The model under review builds one solid part; all positions refer to its coordinate system, in mm. Give positions to 0.01 mm unless a question says otherwise; leave off trailing zeros. Order: outer loops, then holes, each group sorted by start corner. A loop starts at its lowest first (then second) coordinate and runs counter-clockwise, first axis right, second up. Notation, with made-up numbers: (-30.75, 36.25) -> (14.25, 36.25) arc R31 ccw to (14.25, 72.25) -> close; hole circle Ø7 at (19.5, 5.5). An arc over 180 degrees is marked (long way). Use one line per item in the form item = value.
```python
from build123d import *

# Parameters (mm, degrees)
SKETCH1_W                                    = 76
SKETCH1_H                                    = 20
EXTRUDE1_DEPTH                               = 1.5
SKETCH3_W                                    = 15.5
SKETCH3_H                                    = 1.5
SKETCH4_W                                    = 12
SKETCH4_H                                    = 1.5
SKETCH2_W                                    = 12
SKETCH2_H                                    = 1.5
CSK_FOR_M3_COUNTERSUNK_FLAT_HEAD_SCR_2_COUNT = 2
CSK_FOR_M3_COUNTERSUNK_FLAT_HEAD_SCR_2_PITCH = 28.408845453
CSK_FOR_M3_COUNTERSUNK_FLAT_HEAD_SCR_3_COUNT = 2
CSK_FOR_M3_COUNTERSUNK_FLAT_HEAD_SCR_3_PITCH = 56.5


with BuildPart() as part:
    # Sketch1 → Extrude1 (new body)
    with BuildSketch(Plane.XY):
        Rectangle(SKETCH1_W, SKETCH1_H)
    extrude(amount=EXTRUDE1_DEPTH)

    # Sweep1: sweep along a path in Sketch5
    with BuildLine(Plane(origin=(0, 0, 0), x_dir=(0, 0, -1), z_dir=(1, 0, 0))) as sweep1_path:
        Line((-0.75, -10), (-0.75, -13.45))
        ThreePointArc((-0.75, -13.45), (-5.089163608, -14.70129059), (-2.082534588, -11.331683655))
    # Sketch3 → Sweep1 (sweep)
    with BuildSketch(Plane.XZ.offset(10)):
        with Locations((0, 0.75)):
            Rectangle(SKETCH3_W, SKETCH3_H)
    sweep(path=sweep1_path.line)

    # Sweep2: sweep along a path in Sketch7
    with BuildLine(Plane(origin=(32, 0, 0), x_dir=(0, 0, -1), z_dir=(1, 0, 0))) as sweep2_path:
        Line((-0.75, -10), (-0.75, -13.45))
        ThreePointArc((-0.75, -13.45), (-5.089163608, -14.70129059), (-2.082534588, -11.331683655))
    # Sketch4 → Sweep2 (sweep)
    with BuildSketch(Plane.XZ.offset(10)):
        with Locations((32, 0.75)):
            Rectangle(SKETCH4_W, SKETCH4_H)
    sweep(path=sweep2_path.line)

    # Sweep3: sweep along a path in Sketch6
    with BuildLine(Plane(origin=(-32, 0, 0), x_dir=(0, 0, -1), z_dir=(1, 0, 0))) as sweep3_path:
        Line((-0.75, -10), (-0.75, -13.45))
        ThreePointArc((-0.75, -13.45), (-5.089163608, -14.70129059), (-2.082534588, -11.331683655))
    # Sketch2 → Sweep3 (sweep)
    with BuildSketch(Plane.XZ.offset(10)):
        with Locations((-32, 0.75)):
            Rectangle(SKETCH2_W, SKETCH2_H)
    sweep(path=sweep3_path.line)

    # Sketch9 → CSK for M3 Countersunk Flat Head Screw1 (revolve, cut)
    with BuildSketch(Plane(origin=(28.25, -0.25, 1.5), x_dir=(0, -1, 0), z_dir=(1, 0, 0))):
        Polygon((0, 0), (0, 1.50005), (1.6, 1.50005), (1.6, 1.55), (3.15, 0), align=None)
    csk_for_m3_countersunk_flat_head_screw1 = revolve(axis=Axis((28.25, -0.25, 7.85), (0, 0, -1)), mode=Mode.SUBTRACT)

    # CSK for M3 Countersunk Flat Head Scr 2: CSK for M3 Countersunk Flat Head Screw1 ×2
    with Locations(*[Vector(-0.994408591727349, 0.10560091239582468, 0) * (i * CSK_FOR_M3_COUNTERSUNK_FLAT_HEAD_SCR_2_PITCH) for i in range(1, CSK_FOR_M3_COUNTERSUNK_FLAT_HEAD_SCR_2_COUNT)]):
        add(csk_for_m3_countersunk_flat_head_screw1, mode=Mode.SUBTRACT)

    # CSK for M3 Countersunk Flat Head Scr 3: CSK for M3 Countersunk Flat Head Screw1 ×2
    with Locations(*[(-i * CSK_FOR_M3_COUNTERSUNK_FLAT_HEAD_SCR_3_PITCH, 0, 0) for i in range(1, CSK_FOR_M3_COUNTERSUNK_FLAT_HEAD_SCR_3_COUNT)]):
        add(csk_for_m3_countersunk_flat_head_screw1, mode=Mode.SUBTRACT)


solid = part.part
```
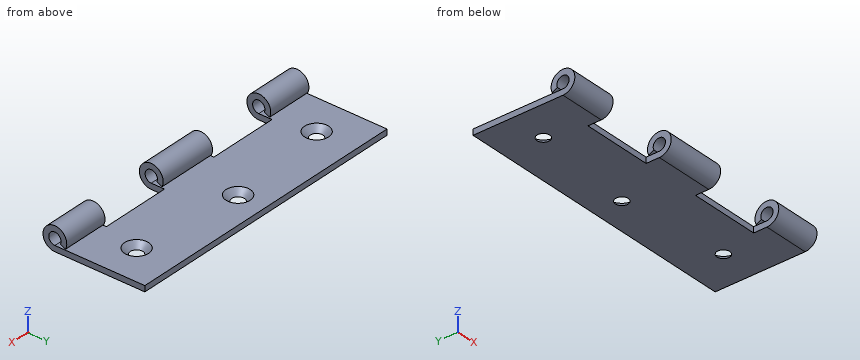
1. Add section B-B on z = 3.1. Give the boundary of the cut face in (x, y).
Values:
outline = (-38, -16.55) -> (-26, -16.55) -> (-26, -15.05) -> (-38, -15.05) -> close; (-38, -11.85) -> (-26, -11.85) -> (-26, -10.35) -> (-38, -10.35) -> close; (-7.75, -16.55) -> (7.75, -16.55) -> (7.75, -15.05) -> (-7.75, -15.05) -> close; (-7.75, -11.85) -> (7.75, -11.85) -> (7.75, -10.35) -> (-7.75, -10.35) -> close; (26, -16.55) -> (38, -16.55) -> (38, -15.05) -> (26, -15.05) -> close; (26, -11.85) -> (38, -11.85) -> (38, -10.35) -> (26, -10.35) -> close
2. Add section D-D on y = 7. Give the boundary of the cut face in (x, z).
Values:
outline = (-38, 0) -> (38, 0) -> (38, 1.5) -> (-38, 1.5) -> close
3. Add section C-C on y = -12.75. Give the boundary of the cut face in (x, z).
Values:
outline = (-38, 0) -> (-26, 0) -> (-26, 1.5) -> (-38, 1.5) -> close; (-38, 4.54) -> (-26, 4.54) -> (-26, 6.12) -> (-38, 6.12) -> close; (-7.75, 0) -> (7.75, 0) -> (7.75, 1.5) -> (-7.75, 1.5) -> close; (-7.75, 4.54) -> (7.75, 4.54) -> (7.75, 6.12) -> (-7.75, 6.12) -> close; (26, 0) -> (38, 0) -> (38, 1.5) -> (26, 1.5) -> close; (26, 4.54) -> (38, 4.54) -> (38, 6.12) -> (26, 6.12) -> close
4. For L1, parallel to X at y = -12.5, z = 1; L2, parallel to Z at x = 31.75, y = -13.45; L3, parallel to Y at x = -34, z = 3.1, list the stretches that pass through material, from the lowest coordinate up.
Values:
L1 = -38 to -26, -7.75 to 7.75, 26 to 38
L2 = 0 to 1.5, 4.7 to 6.2
L3 = -16.55 to -15.05, -11.85 to -10.35
5. For pin 1 Ø4 at (x, y) = (-21.5, -2.5) entering from +Z; pin 2 Ø0.8 at (x, z) = (14.5, 0.5) entering from -Y, all flat-tipped, find the tip position at first contact; note any pin that passes through.
Values:
pin_1 = 1.5
pin_2 = -10
6. Add section A-A on x = 28.25. Give the boundary of the cut face in (y, z), then the cut area to 3 significant figures.
Values:
outline = (-13.45, 0) -> (-1.9, 0) -> (-3.4, 1.5) -> (-13.45, 1.5) arc R1.6 cw (long way) to (-12.01, 2.41) -> (-10.66, 1.76) arc R3.1 ccw (long way) to start; (1.4, 0) -> (10, 0) -> (10, 1.5) -> (2.9, 1.5) -> close
area = 46.2 mm^2
